Here's how the part is built. I have some questions about the finished solid (model axes, mm). Coordinates: 2 decimals unless noted, no trailing zeros. Write each loop counter-clockwise with the first axis right and the second up, starting at its lowest first coordinate (ties: lowest second). Pieces come first, ordered by that corner, then holes.
```python
from build123d import *

# Parameters (mm, degrees)
SKETCH1_R            = 29.25
EXTRUDE_3_8_DEPTH    = 9.525
CUT_EXTRUDE1_DEPTH   = 9.525
SKETCH3_R            = 2.2
M4_THROUGH_DEPTH     = 9.525
SKETCH4_R            = 4.1275
F_3_8_16_DRILL_DEPTH = 9.525
SKETCH6_W            = 18.02935576
SKETCH6_H            = 57.579918791
CUT_EXTRUDE2_DEPTH   = 9.525


with BuildPart() as part:
    # Sketch1 → 3/8 (new body)
    with BuildSketch(Plane.XY):
        with Locations(Location((0, 0, 0), (0, 0, 180))):
            Circle(SKETCH1_R)
    extrude(amount=EXTRUDE_3_8_DEPTH)

    # Sketch2 → Cut-Extrude1 (cut)
    with BuildSketch(Plane.XY.offset(9.525)):
        with BuildLine():
            Line((-3, 24.219267124), (-3, 18.154700472))
            ThreePointArc((-3, 18.154700472), (-3.409072822, 16.942697702), (-4.468950714, 16.226492325))
            ThreePointArc((-4.468950714, 16.226492325), (-5.859541661, 15.777716729), (-7.205966503, 15.210017108))
            ThreePointArc((-7.205966503, 15.210017108), (-9.131700947, 15.327380042), (-10.062257748, 17.017436623))
            Line((-10.062257748, 17.017436623), (-10.062257748, 23.378898605))
            ThreePointArc((-10.062257748, 23.378898605), (-9.690760884, 24.539922954), (-8.714280211, 25.269630397))
            ThreePointArc((-8.714280211, 25.269630397), (-7.073918129, 25.776977757), (-5.404367165, 26.177962402))
            ThreePointArc((-5.404367165, 26.177962402), (-3.736816389, 25.769869318), (-3, 24.219267124))
        make_face()
        with BuildLine():
            Line((-3, 10.72213294), (-3, 7.483314774))
            ThreePointArc((-3, 7.483314774), (-3.236165793, 6.540505732), (-3.888888889, 5.820355935))
            ThreePointArc((-3.888888889, 5.820355935), (-5.257283867, 4.621792546), (-6.270644915, 3.111111111))
            ThreePointArc((-6.270644915, 3.111111111), (-8.518752181, 2.052793582), (-10.062257748, 4))
            Line((-10.062257748, 4), (-10.062257748, 8.658183111))
            ThreePointArc((-10.062257748, 8.658183111), (-9.896091132, 9.45634044), (-9.425202627, 10.121870666))
            ThreePointArc((-9.425202627, 10.121870666), (-7.729958395, 11.468847089), (-5.845262531, 12.534736386))
            ThreePointArc((-5.845262531, 12.534736386), (-3.925412885, 12.408923541), (-3, 10.72213294))
        make_face()
        with BuildLine():
            Line((3, 10.72213294), (3, 7.483314774))
            ThreePointArc((3, 7.483314774), (3.236165793, 6.540505732), (3.888888889, 5.820355935))
            ThreePointArc((3.888888889, 5.820355935), (5.257283867, 4.621792546), (6.270644915, 3.111111111))
            ThreePointArc((6.270644915, 3.111111111), (8.518752181, 2.052793582), (10.062257748, 4))
            Line((10.062257748, 4), (10.062257748, 8.658183111))
            ThreePointArc((10.062257748, 8.658183111), (9.896091132, 9.45634044), (9.425202627, 10.121870666))
            ThreePointArc((9.425202627, 10.121870666), (7.729958395, 11.468847089), (5.845262531, 12.534736386))
            ThreePointArc((5.845262531, 12.534736386), (3.925412885, 12.408923541), (3, 10.72213294))
        make_face()
        with BuildLine():
            Line((3, 24.219267124), (3, 18.154700472))
            ThreePointArc((3, 18.154700472), (3.409072822, 16.942697702), (4.468950714, 16.226492325))
            ThreePointArc((4.468950714, 16.226492325), (5.859541661, 15.777716729), (7.205966503, 15.210017108))
            ThreePointArc((7.205966503, 15.210017108), (9.131700947, 15.327380042), (10.062257748, 17.017436623))
            Line((10.062257748, 17.017436623), (10.062257748, 23.378898605))
            ThreePointArc((10.062257748, 23.378898605), (9.690760884, 24.539922954), (8.714280211, 25.269630397))
            ThreePointArc((8.714280211, 25.269630397), (7.073918129, 25.776977757), (5.404367165, 26.177962402))
            ThreePointArc((5.404367165, 26.177962402), (3.736816389, 25.769869318), (3, 24.219267124))
        make_face()
        with BuildLine():
            Line((-3, -10.72213294), (-3, -7.483314774))
            ThreePointArc((-3, -7.483314774), (-3.236165793, -6.540505732), (-3.888888889, -5.820355935))
            ThreePointArc((-3.888888889, -5.820355935), (-5.257283867, -4.621792546), (-6.270644915, -3.111111111))
            ThreePointArc((-6.270644915, -3.111111111), (-8.518752181, -2.052793582), (-10.062257748, -4))
            Line((-10.062257748, -4), (-10.062257748, -8.658183111))
            ThreePointArc((-10.062257748, -8.658183111), (-9.896091132, -9.45634044), (-9.425202627, -10.121870666))
            ThreePointArc((-9.425202627, -10.121870666), (-7.729958395, -11.468847089), (-5.845262531, -12.534736386))
            ThreePointArc((-5.845262531, -12.534736386), (-3.925412885, -12.408923541), (-3, -10.72213294))
        make_face()
        with BuildLine():
            Line((3, -10.72213294), (3, -7.483314774))
            ThreePointArc((3, -7.483314774), (3.236165793, -6.540505732), (3.888888889, -5.820355935))
            ThreePointArc((3.888888889, -5.820355935), (5.257283867, -4.621792546), (6.270644915, -3.111111111))
            ThreePointArc((6.270644915, -3.111111111), (8.518752181, -2.052793582), (10.062257748, -4))
            Line((10.062257748, -4), (10.062257748, -8.658183111))
            ThreePointArc((10.062257748, -8.658183111), (9.896091132, -9.45634044), (9.425202627, -10.121870666))
            ThreePointArc((9.425202627, -10.121870666), (7.729958395, -11.468847089), (5.845262531, -12.534736386))
            ThreePointArc((5.845262531, -12.534736386), (3.925412885, -12.408923541), (3, -10.72213294))
        make_face()
        with BuildLine():
            Line((3, -24.219267124), (3, -18.154700472))
            ThreePointArc((3, -18.154700472), (3.409072822, -16.942697702), (4.468950714, -16.226492325))
            ThreePointArc((4.468950714, -16.226492325), (5.859541661, -15.777716729), (7.205966503, -15.210017108))
            ThreePointArc((7.205966503, -15.210017108), (9.131700947, -15.327380042), (10.062257748, -17.017436623))
            Line((10.062257748, -17.017436623), (10.062257748, -23.378898605))
            ThreePointArc((10.062257748, -23.378898605), (9.690760884, -24.539922954), (8.714280211, -25.269630397))
            ThreePointArc((8.714280211, -25.269630397), (7.073918129, -25.776977757), (5.404367165, -26.177962402))
            ThreePointArc((5.404367165, -26.177962402), (3.736816389, -25.769869318), (3, -24.219267124))
        make_face()
        with BuildLine():
            Line((-3, -24.219267124), (-3, -18.154700472))
            ThreePointArc((-3, -18.154700472), (-3.409072822, -16.942697702), (-4.468950714, -16.226492325))
            ThreePointArc((-4.468950714, -16.226492325), (-5.859541661, -15.777716729), (-7.205966503, -15.210017108))
            ThreePointArc((-7.205966503, -15.210017108), (-9.131700947, -15.327380042), (-10.062257748, -17.017436623))
            Line((-10.062257748, -17.017436623), (-10.062257748, -23.378898605))
            ThreePointArc((-10.062257748, -23.378898605), (-9.690760884, -24.539922954), (-8.714280211, -25.269630397))
            ThreePointArc((-8.714280211, -25.269630397), (-7.073918129, -25.776977757), (-5.404367165, -26.177962402))
            ThreePointArc((-5.404367165, -26.177962402), (-3.736816389, -25.769869318), (-3, -24.219267124))
        make_face()
    extrude(amount=-CUT_EXTRUDE1_DEPTH, mode=Mode.SUBTRACT)

    # Sketch3 → M4_through (cut)
    with BuildSketch(Plane.XY.offset(9.525)):
        with Locations((0, 15)):
            Circle(SKETCH3_R)
        with Locations((0, -15)):
            Circle(SKETCH3_R)
    extrude(amount=-M4_THROUGH_DEPTH, mode=Mode.SUBTRACT)

    # Sketch4 → 3/8_-16-DRILL (cut)
    with BuildSketch(Plane.XY.offset(9.525)):
        Circle(SKETCH4_R)
    extrude(amount=-F_3_8_16_DRILL_DEPTH, mode=Mode.SUBTRACT)

    # Sketch6 → Cut-Extrude2 (cut)
    with BuildSketch(Plane.XY.offset(9.525)):
        with Locations((-22.076935628, -1.336167669)):
            Rectangle(SKETCH6_W, SKETCH6_H)
        with Locations((22.076935628, -1.336167669)):
            Rectangle(SKETCH6_W, SKETCH6_H)
    extrude(amount=-CUT_EXTRUDE2_DEPTH, mode=Mode.SUBTRACT)


solid = part.part
```
1) Imagine slicing it at B-B on y = 0. Please give me the cut outline in (x, z) (1 decimal).
Values follow:
outline: (-13.1, 0) - (-4.1, 0) - (-4.1, 9.5) - (-13.1, 9.5) - close; (4.1, 0) - (13.1, 0) - (13.1, 9.5) - (4.1, 9.5) - close
2) Will these pins go through, and if not, where does the flat tip stop? pin 1 (1.5 mm diameter, centred on x = -9.5, z = 5.5, fed in from -Y); pin 2 (1 mm diameter, centred on x = -1.5, z = 8.5, fed in from +Y); pin 3 (1 mm diameter, centred on x = 5.5, z = 6.5, fed in from +Y).
Values follow:
pin 1: stops at y = -27.91
pin 2: stops at y = 29.23
pin 3: stops at y = 28.82
3) I need wall thicknesses on probe 1 along Y at (x, z) = (0, 6.75); probe 2 along X at (y, z) = (8.5, 8.5); probe 3 along Y at (x, z) = (-9.5, 2). Which ranges of each line are inside material? Lowest first, please.
Values follow:
probe 1: y = -29.25 to -17.2, -12.8 to -4.13, 4.13 to 12.8, 17.2 to 29.25
probe 2: x = -13.06 to -10.06, -3 to 3, 10.06 to 13.06
probe 3: y = -27.66 to -24.77, -15.63 to -10.05, -2.61 to 2.61, 10.05 to 15.63, 24.77 to 27.66
4) Imagine slicing it at A-A on x = 0. Count the separate pieces of the cut face and the enclosed holes in it, then the cut area to 3 significant figures.
Values follow:
separate pieces: 4
enclosed holes: 0
area: 395 mm2
5) We'd pull the mould along X, two halves only. Please class faces 1 (the face through (5.8, 15.8, 4.8)), 2 (the face through (0, -7, 9.525)), 3 (the face through (0.19, 29.25, 4.7)): pulls with the +X half, pulls with the -X half, needs draft (parallel to the pull), parting line crosses it, or undercut.
Values follow:
face 1: undercut
face 2: needs draft
face 3: parting line crosses it
6) Imagine slicing it at C-C on y = 22.5. Please give me the cut outline in (x, z) (3 decimals).
Values follow:
outline: (-13.062, 0) - (-10.062, 0) - (-10.062, 9.525) - (-13.062, 9.525) - close; (-3, 0) - (3, 0) - (3, 9.525) - (-3, 9.525) - close; (10.062, 0) - (13.062, 0) - (13.062, 9.525) - (10.062, 9.525) - close
